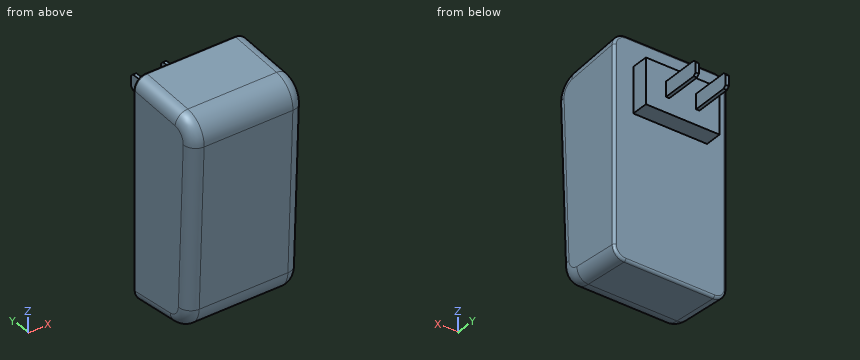
```python
from build123d import *

# Parameters (mm, degrees)
F1_DEPTH = 23.5
F2_W     = 30.75
F2_H     = 18.8
F2_W_2   = 1.4
F2_H_2   = 6.21
F3_DEPTH = 7
F4_DEPTH = 23.5
F5_R     = 10
F6_R     = 5
F7_R     = 1
F8_SIZE  = 1


with BuildPart() as f1:
    # F0 (on Right) → F1 (new body, symmetric)
    with BuildSketch(Plane.YZ):
        Polygon((0, 0), (0, 90.6), (-33.3, 87.7318647873), (-29.8, 2.658541554), align=None)
    extrude(amount=F1_DEPTH, both=True)

    # F2 (on Front) → F3 (join)
    with BuildSketch(Plane.XZ):
        with Locations((0, 69.95)):
            Rectangle(F2_W, F2_H)
        with Locations((-6.265, 69.95)):
            Rectangle(F2_W_2, F2_H_2, mode=Mode.SUBTRACT)
        with Locations((6.265, 69.95)):
            Rectangle(F2_W_2, F2_H_2, mode=Mode.SUBTRACT)
        with Locations((6.265, 69.95)):
            Rectangle(F2_W_2, F2_H_2)
        with Locations((-6.265, 69.95)):
            Rectangle(F2_W_2, F2_H_2)
    extrude(amount=-F3_DEPTH)

    # F2 (on Front) → F4 (join)
    with BuildSketch(Plane.XZ):
        with Locations((-6.265, 69.95)):
            Rectangle(F2_W_2, F2_H_2)
        with Locations((6.265, 69.95)):
            Rectangle(F2_W_2, F2_H_2)
    extrude(amount=-F4_DEPTH)

    # F5
    f5_edges = [f1.edges().sort_by_distance(p)[0] for p in [
        (0, -33.3, 87.731865),
        (0, -29.8, 2.658542),
    ]]
    fillet(f5_edges, radius=F5_R)

    # F6
    f6_edges = [f1.edges().sort_by_distance(p)[0] for p in [
        (23.5, -31.533869, 44.803107),
        (-23.5, -31.533869, 44.803107),
    ]]
    fillet(f6_edges, radius=F6_R)

    # F7
    f7_edges = [f1.edges().sort_by_distance(p)[0] for p in [
        (23.5, 0, 45.300673),
    ]]
    fillet(f7_edges, radius=F7_R)

    # F8
    f8_edges = [f1.edges().sort_by_distance(p)[0] for p in [
        (-6.265, 23.5, 73.055),
        (-6.265, 23.5, 66.845),
        (6.265, 23.5, 73.055),
        (6.265, 23.5, 66.845),
    ]]
    chamfer(f8_edges, length=F8_SIZE)


solid = f1.part
```
Check sheet for the modelled part. Datum: model origin and axes. Units: mm. Round coordinates to 2 decimals unless told otherwise and drop trailing zeros. Loops run counter-clockwise (first coordinate to the right, second up) from the corner with the lowest first, then second, coordinate; pieces in that order, holes last. Notation, with made-up numbers: (38, 42) - (88, 42) arc R18 ccw to (88, 50) - close; hole circle Ø7 at (-8, -5.75). An arc over 180 degrees is marked (long way). Write item = value, one per line. Start each with the question number.
Q1. Section check A-A (x = -1.5). Record the boundary of the cut face in (y, z).
Q2. Thickness scan on L1, parallel to Y at x = 15.5, z = 78.5 (3 decimals); L2, parallel to Z at x = -6, y = 0.5; L3, parallel to Y at x = 21, z = 47.5. Record the ranges inside material, lowest first.
Q3. Depth check by flat-ended pin: P1, Ø4, axis at x = 6, z = 63.5, coming from the +Y side; P2, Ø1.9, axis at y = 12.5, z = 69, coming from the +X side (3 decimals); P3, Ø5, axis at x = -3, y = 16.5, coming from the +Z side; P4, Ø1.1, axis at x = 6.5, y = 14.5, coming from the +Z side (3 decimals). Enter the tip coordinate at first touch or a pass-through.
Derived:
q1.outline = (-32.91, 78.18) - (-30.16, 11.43) arc R10 ccw to (-21.06, 1.88) - (-1.09, 0.1) arc R1 ccw to (0, 1.09) - (0, 60.55) - (7, 60.55) - (7, 79.35) - (0, 79.35) - (0, 89.51) arc R1 ccw to (-1.09, 90.51) - (-23.77, 88.55) arc R10 ccw to start
q2.L1 = -32.915 to 0
q2.L2 = 60.55 to 79.35
q2.L3 = -30.97 to 0
q3.P1 = 7
q3.P2 = 6.965
q3.P3 = through
q3.P4 = 73.055
